Could you check a few things on this model? Use its own coordinates, in mm. A direction names the side the tool comes from. Give positions to 0.01 mm unless a question says otherwise; leave off trailing zeros. Order: outer loops, then holes, each group sorted by start corner. A loop starts at its lowest first (then second) coordinate and runs counter-clockwise, first axis right, second up.
(1) If we mould it in two halves opening along X, with no side actions, what happens to faces 4 (the flat face through (-40, -35, 4)), 5 (the cylindrical face through (-38, -35, 4)), 6 (the flat face through (-26.5, -6.2, 8))? For each: released by +X, released by -X, zero draft, split by the parting line, or undercut.
(2) Imagine slicing it at D-D, the plane x = 0. Write out the boundary of the cut face in (y, z).
(3) Imagine slicing it at A-A, the plane y = -25. Write out the boundary of the cut face in (x, z).
(4) Imagine slicing it at C-C, the plane x = -36. Write out the boundary of the cut face in (y, z), then the cut area to 3 significant figures.
(5) Will these pins go through, and if not, where does the flat tip stop? pin 1 (1.5 mm diameter, centred on y = -20, z = 2, fed in from -X); pin 2 (2.5 mm diameter, centred on y = -18.5, z = 3.5, fed in from +X); pin 3 (3 mm diameter, centred on x = 36, z = 4, fed in from +Y); pin 4 (4 mm diameter, centred on y = 15, z = 5.5, fed in from +X).
(6) Imagine slicing it at B-B, the plane z = 4. Write out the boundary of the cut face in (x, y), then the cut area to 3 significant figures.
(7) If I drill on probe 1 along X at (y, z) = (-35.2, 4); probe 2 along X at (y, z) = (-12, 0.5); probe 3 along Y at (x, z) = (-31.5, 6.5), over which ranges is the centre line in solid material (lowest first)?
(8) On a 3-axis mill with a long thin cutter (end or side, diameter ignored), from which of +Z, -Z, +X, -X, +Y, -Y can I reach the whole of each face in a straight line? I mean faces 1 (the flat face through (28, -17, 4)), 2 (the flat face through (26, -18, 4)), 3 (the flat face through (-28, -17, 4)). Say none if no direction works.
from build123d import *

# Parameters (mm, degrees)
BOSS_EXTRUDE1_DEPTH         = 8
TAP_DRILL_FOR_M4X0_7_TAP1_D = 3.3
SKETCH4_R                   = 2
CUT_EXTRUDE1_DEPTH          = 75.215901261


with BuildPart() as part:
    # Sketch3 → Boss-Extrude1 (new body)
    with BuildSketch(Plane.XY):
        with BuildLine():
            Line((28, 0), (28, -34))
            Line((28, -34), (40, -34))
            Line((40, -34), (40, -36))
            Line((40, -36), (26, -36))
            Line((26, -36), (26, 0))
            ThreePointArc((26, 0), (0, 26), (-26, 0))
            Line((-26, 0), (-26, -36))
            Line((-26, -36), (-40, -36))
            Line((-40, -36), (-40, -34))
            Line((-40, -34), (-28, -34))
            Line((-28, -34), (-28, 0))
            ThreePointArc((-28, 0), (0, 28), (28, 0))
        make_face()
    extrude(amount=BOSS_EXTRUDE1_DEPTH)

    # Tap Drill for M4x0.7 Tap1 (through all)
    with Locations(Plane(origin=(0, -34, 0), x_dir=(1, 0, 0), z_dir=(0, 1, 0))):
        with Locations((-36, -4), (36, -4)):
            Hole(TAP_DRILL_FOR_M4X0_7_TAP1_D / 2)

    # Sketch4 → Cut-Extrude1 (cut, through all)
    with BuildSketch(Plane(origin=(0, -34, 0), x_dir=(1, 0, 0), z_dir=(0, 1, 0))):
        with Locations(Location((-36, -4, 0), (0, 0, 270))):
            Circle(SKETCH4_R)
        with Locations(Location((36, -4, 0), (0, 0, 270))):
            Circle(SKETCH4_R)
    extrude(amount=-CUT_EXTRUDE1_DEPTH, mode=Mode.SUBTRACT)


solid = part.part
Answer block:
1. face 4: released by -X
1. face 5: undercut
1. face 6: zero draft
2. outline: (26, 0) - (28, 0) - (28, 8) - (26, 8) - close
3. outline: (-28, 0) - (-26, 0) - (-26, 8) - (-28, 8) - close; (26, 0) - (28, 0) - (28, 8) - (26, 8) - close
4. outline: (-36, 0) - (-34, 0) - (-34, 2) - (-36, 2) - close; (-36, 6) - (-34, 6) - (-34, 8) - (-36, 8) - close
4. area: 8.00 mm2
5. pin 1: stops at x = -28
5. pin 2: stops at x = 28
5. pin 3: passes through
5. pin 4: stops at x = 24.8
6. outline: (-40, -36) - (-38, -36) - (-38, -34) - (-40, -34) - close; (-34, -36) - (-26, -36) - (-26, 0) arc R26 cw to (26, 0) - (26, -36) - (34, -36) - (34, -34) - (28, -34) - (28, 0) arc R28 ccw to (-28, 0) - (-28, -34) - (-34, -34) - close; (38, -36) - (40, -36) - (40, -34) - (38, -34) - close
6. area: 346 mm2
7. probe 1: x = -40 to -38, -34 to -26, 26 to 34, 38 to 40
7. probe 2: x = -28 to -26, 26 to 28
7. probe 3: y = -36 to -34
8. face 1: +Z, -Z, +X, +Y
8. face 2: +Z, -Z, -Y
8. face 3: +Z, -Z, -X, +Y
